from build123d import *

# Parameters (mm, degrees)
F0_R     = 17.5
F1_DEPTH = 2.5
F2_R     = 17.5
F3_DEPTH = 50
F3_TAPER = 15
F4_R     = 3.6137849114
F5_DEPTH = 60
F6_R     = 13.2346261553


# Not quite as in the source:
# - an extrude whose draft closes it to a point is written as a loft to that point


with BuildPart() as f1:
    # F0 (on Top) → F1 (new body)
    with BuildSketch(Plane.XY):
        with BuildLine():
            Line((0, 38.8068709316), (-35.2930977718, 38.8068709316))
            ThreePointArc((-35.2930977718, 38.8068709316), (-38.8286316778, 37.3424048375), (-40.2930977718, 33.8068709316))
            Line((-40.2930977718, 33.8068709316), (-40.2930977718, 0))
            ThreePointArc((-40.2930977718, 0), (-38.8286316778, -3.5355339059), (-35.2930977718, -5))
            Line((-35.2930977718, -5), (0, -5))
            ThreePointArc((0, -5), (3.5355339059, -3.5355339059), (5, 0))
            Line((5, 0), (5, 33.8068709316))
            ThreePointArc((5, 33.8068709316), (3.5355339059, 37.3424048375), (0, 38.8068709316))
        make_face()
        with Locations((-17.6465488859, 16.9034354658)):
            Circle(F0_R, mode=Mode.SUBTRACT)
        with Locations((-17.6465488859, 16.9034354658)):
            Circle(F0_R)
    extrude(amount=F1_DEPTH)

    # F2 (on face) → F3 (join)
    with BuildSketch(Plane.XY.offset(2.5)):
        with Locations((-17.6465488859, 16.9034354658)):
            Circle(F2_R)
    extrude(amount=F3_DEPTH, taper=F3_TAPER)

    # F4 (on Right) → F5 (cut)
    with BuildSketch(Plane.YZ):
        with Locations((17.7631601691, 42.927633971)):
            Circle(F4_R)
    extrude(amount=-F5_DEPTH, mode=Mode.SUBTRACT)

    # F6 (on face) → F7 section 0
    with BuildSketch(Plane(origin=(0, 0, 0), x_dir=(1, 0, 0), z_dir=(0, 0, -1)), mode=Mode.PRIVATE) as f7_s0:
        with Locations((-17.6465488859, -16.9034354658)):
            Circle(F6_R)
    loft([f7_s0.sketch, Vertex(-17.6465488859, 16.9034354658, 22.9230449201)], ruled=True, mode=Mode.SUBTRACT)


solid = f1.part
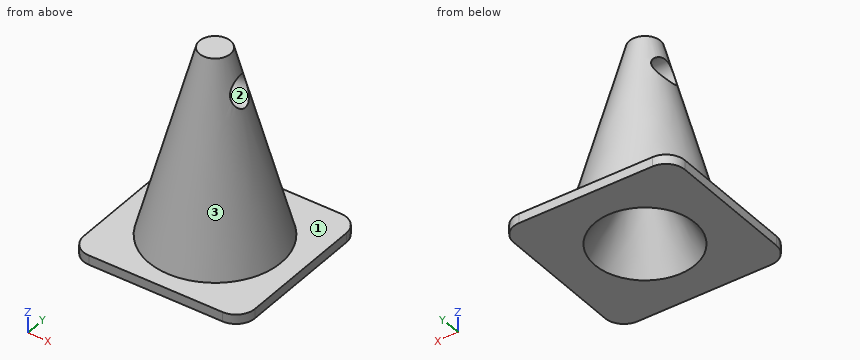
Source: CAD feature listing. Evaluate the final solid. Frame: model axes, mm. Face numbers are marked on the shaded views. Coordinates: 2 decimals unless noted, no trailing zeros. Order: outer loops, then holes, each group sorted by start corner. A loop starts at its lowest first (then second) coordinate and runs counter-clockwise, first axis right, second up.
Item 1: First-contact query: P1, Ø8, axis at x = -10, y = 17, coming from the -Z side; P2, Ø6, axis at y = 17.76, z = 42.93, coming from the +X side; P3, Ø10, axis at x = -3, y = 26, coming from the -Z side; P4, Ø2, axis at x = -21.5, y = 19.5, coming from the -Z side. Flat tips, straight axial feed; report the tip coordinate or a pass-through.
Output values:
P1: stops at z = 2.75
P2: passes through
P3: stops at z = 0
P4: stops at z = 13.14
Item 2: Cut plane B-B (y = -2). Return loops of the section in (x, z), plus the area to 3 significant figures.
Output values:
outline: (-39.88, 0) - (4.58, 0) - (4.58, 2.5) - (-39.88, 2.5) - close
area: 111 mm2
Item 3: Material intervals for line 1 (Z direction, x = 2, y = 10); line 2 (Y direction, x = -13.5, z = 16); line 3 (Y direction, x = -27.5, z = 4), sorted ascending.
Output values:
line 1: z = 0 to 2.5
line 2: y = 3.65 to 30.15
line 3: y = 2.93 to 12.18, 21.62 to 30.88
Item 4: Cut plane D-D (z = 26.5). Return loops of the section in (x, y), plus the area to 3 significant figures.
Output values:
outline: circle Ø22.14 at (-17.65, 16.9)
area: 385 mm2
Item 5: Pull-direction query (Y, two-part tool) for the marked faces 1, 2 and 3; classes: pulls with the +Y half, pulls with the -Y half, needs draft (parallel to the pull), parting line crosses it, or undercut.
Output values:
face 1: needs draft
face 2: undercut
face 3: parting line crosses it
Item 6: Cut plane C-C (x = -36.5). Return loops of the section in (y, z), plus the area to 3 significant figures.
Output values:
outline: (-4.85, 0) - (38.66, 0) - (38.66, 2.5) - (-4.85, 2.5) - close
area: 109 mm2
Item 7: Cut plane A-A (z = 16.5). Return loops of the section in (x, y), plus the area to 3 significant figures.
Output values:
outline: circle Ø27.5 at (-17.65, 16.9); hole circle Ø7.42 at (-17.65, 16.9)
area: 551 mm2
